Work out the finished part from the listing and answer in its coordinate system (mm). A direction names the side the tool comes from. Coordinates: 2 decimals unless noted, no trailing zeros. Write each loop counter-clockwise with the first axis right and the second up, starting at its lowest first coordinate (ties: lowest second). Pieces come first, ordered by that corner, then holes. Notation, with made-up numbers: (2, 15.25) - (46, 15.25) arc R35 ccw to (46, 47.25) - close; hole circle Ø2 at (-2, 79). An arc over 180 degrees is marked (long way). One line per item, written item: value.
```python
from build123d import *

# Parameters (mm, degrees)
SKETCH_W        = 100
SKETCH_H        = 160
PAD_DEPTH       = 26
SKETCH001_W     = 96
SKETCH001_H     = 156
PAD001_DEPTH    = 28
SKETCH005_W     = 92
SKETCH005_H     = 152
POCKET_DEPTH    = 24
SKETCH003_R     = 9
POCKET001_DEPTH = 28.001
SKETCH002_R     = 1
POCKET002_DEPTH = 28.001
SKETCH006_W     = 96
SKETCH006_H     = 156
POCKET003_DEPTH = 2
SKETCH007_R     = 1.5
POCKET004_DEPTH = 10


with BuildPart() as part:
    # Sketch → Pad (new body)
    with BuildSketch(Plane.XY):
        Rectangle(SKETCH_W, SKETCH_H)
    extrude(amount=PAD_DEPTH)

    # Sketch001 → Pad001 (join)
    with BuildSketch(Plane.XY):
        Rectangle(SKETCH001_W, SKETCH001_H)
    extrude(amount=PAD001_DEPTH)

    # Sketch005 → Pocket (cut)
    with BuildSketch(Plane.XY.offset(28)):
        Rectangle(SKETCH005_W, SKETCH005_H)
    extrude(amount=-POCKET_DEPTH, mode=Mode.SUBTRACT)

    # Sketch003 → Pocket001 (cut, through all)
    with BuildSketch(Plane.XY):
        with Locations((33.25, 36.5)):
            Circle(SKETCH003_R)
        with Locations((25.45, 13.5)):
            Circle(SKETCH003_R)
        with Locations((25.45, -9.5)):
            Circle(SKETCH003_R)
        with Locations((33.25, -32.5)):
            Circle(SKETCH003_R)
        with Locations((-33.25, 36.5)):
            Circle(SKETCH003_R)
        with Locations((-25.45, 13.5)):
            Circle(SKETCH003_R)
        with Locations((-25.45, -9.5)):
            Circle(SKETCH003_R)
        with Locations((-33.25, -32.5)):
            Circle(SKETCH003_R)
    extrude(amount=POCKET001_DEPTH, mode=Mode.SUBTRACT)

    # Sketch002 → Pocket002 (cut, through all)
    with BuildSketch(Plane.XY):
        with Locations((42.25, 72.5)):
            Circle(SKETCH002_R)
        with Locations((-42.25, 72.5)):
            Circle(SKETCH002_R)
        with Locations((42.25, -72.5)):
            Circle(SKETCH002_R)
        with Locations((-42.25, -72.5)):
            Circle(SKETCH002_R)
    extrude(amount=POCKET002_DEPTH, mode=Mode.SUBTRACT)

    # Sketch006 → Pocket003 (cut)
    with BuildSketch(Plane.XY):
        Rectangle(SKETCH006_W, SKETCH006_H)
    extrude(amount=POCKET003_DEPTH, mode=Mode.SUBTRACT)

    # Sketch007 → Pocket004 (cut)
    with BuildSketch(Plane.XZ.offset(80)):
        with Locations((-15, 15)):
            Circle(SKETCH007_R)
        with Locations((-5, 15)):
            Circle(SKETCH007_R)
        with Locations((5, 15)):
            Circle(SKETCH007_R)
        with Locations((15, 15)):
            Circle(SKETCH007_R)
    extrude(amount=-POCKET004_DEPTH, mode=Mode.SUBTRACT)


solid = part.part
```
Item 1: Which of the six approach directions +Z, -Z, +X, -X, +Y, -Y give full straight-line access (tool end or side, diameter ignored) to faces 5 (the face through (-16.5, -78.03, 15.07)), 6 (the face through (18.31, 8.02, 2.99)), 7 (the face through (-1, -76, 16))?
Evaluation:
face 5: -Y
face 6: +Z, -Z
face 7: +Z
Item 2: Section A-A, the plane y = 13.5 is taken. Determine the outline of the cut face in (x, z).
Evaluation:
outline: (-50, 0) - (-48, 0) - (-48, 2) - (-34.45, 2) - (-34.45, 4) - (-46, 4) - (-46, 28) - (-48, 28) - (-48, 26) - (-50, 26) - close; (-16.45, 2) - (16.45, 2) - (16.45, 4) - (-16.45, 4) - close; (34.45, 2) - (48, 2) - (48, 0) - (50, 0) - (50, 26) - (48, 26) - (48, 28) - (46, 28) - (46, 4) - (34.45, 4) - close
Item 3: Section C-C, the plane x = 9 is taken. Determine the outline of the cut face in (y, z), then the cut area to 3 significant figures.
Evaluation:
outline: (-80, 0) - (-78, 0) - (-78, 2) - (78, 2) - (78, 0) - (80, 0) - (80, 26) - (78, 26) - (78, 28) - (76, 28) - (76, 4) - (-76, 4) - (-76, 28) - (-78, 28) - (-78, 26) - (-80, 26) - close
area: 512 mm2
Item 4: Determine the mould class of faces 1 (the face through (-48.4, 0.4, 0)), 2 (the face through (6.386, -78.028, 14.425)), 3 (the face through (-50, -1, 13)), 4 (the face through (13.5, -78.03, 15.07)) for opening direction Z: +Z half, -Z half, draft (parallel to the pull), parting line (faces both ways), or undercut.
Evaluation:
face 1: -Z half
face 2: undercut
face 3: draft
face 4: undercut
Item 5: Section B-B, the plane z = 20.5 is taken. Determine the outline of the cut face in (x, y).
Evaluation:
outline: (-50, -80) - (50, -80) - (50, 80) - (-50, 80) - close; hole (-46, -76) - (46, -76) - (46, 76) - (-46, 76) - close
Item 6: Consider probe 1 along X at (y, z) = (-72.5, 2.7); probe 2 along X at (y, z) = (13.5, 2.9); probe 3 along Y at (x, z) = (-27, 7.75). Determine where each line is inside the solid, lowest interval first.
Evaluation:
probe 1: x = -50 to -43.25, -41.25 to 41.25, 43.25 to 50
probe 2: x = -50 to -34.45, -16.45 to 16.45, 34.45 to 50
probe 3: y = -80 to -76, 76 to 80
Item 7: Section D-D, the plane y = 53.5 is taken. Determine the outline of the cut face in (x, z).
Evaluation:
outline: (-50, 0) - (-48, 0) - (-48, 2) - (48, 2) - (48, 0) - (50, 0) - (50, 26) - (48, 26) - (48, 28) - (46, 28) - (46, 4) - (-46, 4) - (-46, 28) - (-48, 28) - (-48, 26) - (-50, 26) - close
Item 8: Given pin 1 (11 mm diameter, centred on x = -33.25, y = 36.5, fed in from -Z); pin 2 (1 mm diameter, centred on x = 37, y = -21, fed in from -Z); pin 3 (1.6 mm diameter, centred on y = 0.5, z = 27, fed in from -X), each flat-ended and moving along its own axis, determine where each tip first touches the part or whether it passes through.
Evaluation:
pin 1: passes through
pin 2: stops at z = 2
pin 3: stops at x = -48
